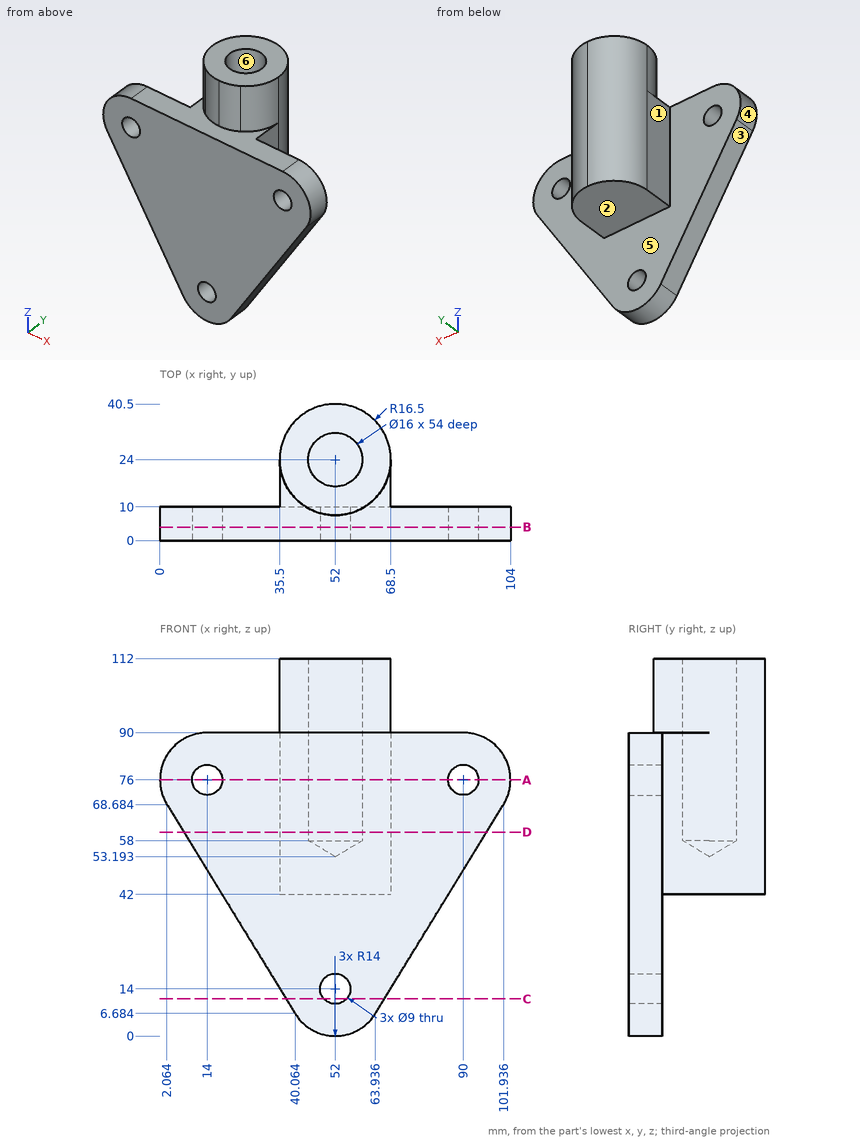
Study the drawing (mm; zero at the part's minimum x, y, z) and answer. A direction names the side the tool comes from. Coordinates: 2 decimals unless noted, no trailing zeros. Write each loop counter-clockwise with the first axis right and the second up, starting at its lowest first coordinate (ties: lowest second). Pieces come first, ordered by that corner, then holes. Notation, with made-up numbers: M -23.5,-27.75 L -4.5,-27.75 A20 cw -4.5,-13.75 Z; hole C 40.5,0 d3. An arc over 180 degrees is marked long. Use a Markdown table: item, result. Add a question column.
1. Section B-B (y = 4) is taken. Give the vertices of the cut face in (x, z).
2. Which of the six approach directions +Z, -Z, +X, -X, +Y, -Y give full straight-line access (tool end or side, diameter ignored) to the marked faces 1, 2 and 3?
3. Straight lines are drawn through the part: line 1 along X through (y, z) = (24, 78); line 2 along Z through (x, y) = (52.5, 3.5); line 3 along Y through (x, z) = (52, 83). For each, find the intervals that lie inside material, in ascending order. Write a range as [from, to].
4. For a pull along X with two mould halves and no side action, classify the marked faces 4, 5 and 6 as +X half, -X half, draft (parallel to the pull), parting line (faces both ways), or undercut.
5. Section C-C (z = 11) is taken. Give the vertices of the cut face in (x, y).
6. Given P1, Ø15, axis at x = 45, y = 23.5, coming from the -Z side; P2, Ø12, axis at x = 42, z = 33, coming from the +Y side; P3, Ø1.5, axis at y = 29, z = 84.5, coming from the -X side, each flat-ended and moving along its own axis, determine where each tip first touches the part or whether it passes through.
7. Section A-A (z = 76) is taken. Give the vertices of the cut face in (x, y).
8. Section D-D (z = 60.5) is taken. Give the vertices of the cut face in (x, y), plus the area to 3 significant figures.
Data:
| question | item | result |
|---|---|---|
| 1 | outline | M 2.06,68.68 L 40.06,6.68 A14 ccw 63.94,6.68 L 101.94,68.68 A14 ccw 90,90 L 14,90 A14 ccw Z; hole C 14,76 d9; hole C 52,14 d9; hole C 90,76 d9 |
| 2 | face 1 | +Z, -Z, -X, +Y |
| 2 | face 2 | -Z, +X, -X, +Y |
| 2 | face 3 | -Z, -X, +Y, -Y |
| 3 | line 1 | x = [35.5, 44], [60, 68.5] |
| 3 | line 2 | z = [0.01, 9.53], [18.47, 90] |
| 3 | line 3 | y = [0, 16], [32, 40.5] |
| 4 | face 4 | -X half |
| 4 | face 5 | draft |
| 4 | face 6 | undercut |
| 5 | outline | M 37.42,0 L 48.65,0 L 48.65,10 L 37.42,10 Z; M 55.35,0 L 66.58,0 L 66.58,10 L 55.35,10 Z |
| 6 | P1 | stops at z = 42 |
| 6 | P2 | stops at y = 10 |
| 6 | P3 | stops at x = 36.06 |
| 7 | outline | M 0,0 L 9.5,0 L 9.5,10 L 0,10 Z; M 18.5,0 L 85.5,0 L 85.5,10 L 68.5,10 L 68.5,24 A16.5 ccw 35.5,24 L 35.5,10 L 18.5,10 Z; M 94.5,0 L 104,0 L 104,10 L 94.5,10 Z; hole C 52,24 d16 |
| 8 | outline | M 7.08,0 L 96.92,0 L 96.92,10 L 68.5,10 L 68.5,24 A16.5 ccw 35.5,24 L 35.5,10 L 7.08,10 Z; hole C 52,24 d16 |
| 8 | area | 1,590 mm2 |
